Autodesk Inventor part; units mm, degrees
ref_plane "YZ Plane" through (0, 0, 0) normal (1, 0, 0) x (0, 1, 0)
ref_plane "XZ Plane" through (0, 0, 0) normal (0, 1, 0) x (-1, 0, 0)
ref_plane "XY Plane" through (0, 0, 0) normal (0, 0, 1) x (1, 0, 0)
sketch "Sketch1" plane through (0, 0, 0) normal (0, 0, 1) x (1, 0, 0)
  line L0 (17.35, -13.5) -> (-17.35, -13.5)
  line L1 (-17.35, -13.5) -> (-17.35, 13.5)
  line L2 (-17.35, 13.5) -> (17.35, 13.5)
  line L3 (17.35, 13.5) -> (17.35, -13.5)
  line L4 (17.35, -13.5) -> (-17.35, 13.5) construction
  line L5 (-17.35, -13.5) -> (17.35, 13.5) construction
  point P0 (0, 0)
  dimension "d0" = 27
  dimension "d1" = 34.7
extrude "Extrusion1" add sketch "Sketch1" along normal blind 10
sketch "Sketch2" plane through (0, 0, 10) normal (0, 0, 1) x (1, 0, 0)
  line L0 (17.35, -6) -> (-17.35, -6)
  line L1 (-17.35, -6) -> (-17.35, 6)
  line L2 (-17.35, 6) -> (17.35, 6)
  line L3 (17.35, 6) -> (17.35, -6)
  line L4 (17.35, -6) -> (-17.35, 6) construction
  line L5 (-17.35, -6) -> (17.35, 6) construction
  point P0 (0, 0)
  point P1 (17.35, 13.5)
  dimension "d4" = 12
extrude "Extrusion2" cut sketch "Sketch2" against normal blind 5
sketch "Sketch3" plane through (0, 0, 0) normal (0, 0, -1) x (-1, 0, 0)
  point P0 (0, 0)
  point P1 (-7.5, 10)
  point P2 (-7.5, -10)
  point P3 (7.5, 10)
  point P4 (7.5, -10)
  dimension "d7" = 20
  dimension "d8" = 10
  dimension "d9" = 15
  dimension "d10" = 7.5
hole "Hole1" at (7.5, 10, 0) at (7.5, -10, 0) at (-7.5, 10, 0) at (-7.5, -10, 0) direction (0, 0, 1) diameter 2.459 depth 8.8 tip angle 118
properties part number "MGN12C" material "Stainless Steel"
CAD build for the part. Positions are in the model's coordinates, mm. A direction names the side the tool comes from. Round coordinates to 2 decimals unless told otherwise and drop trailing zeros. Order: outer loops, then holes, each group sorted by start corner. A loop starts at its lowest first (then second) coordinate and runs counter-clockwise, first axis right, second up. Notation, with made-up numbers: M 31.25,-33.75 L 61.25,-33.75 A22 cw 61.25,-17.75 Z; hole C 10.5,56 d3. An arc over 180 degrees is marked long. Use one line per item in the form item = value.
Q1. Which spindle directions (+Z, -Z, +X, -X, +Y, -Y) get a long thin tool onto all of the face, cutting with end or side? Do faces 1 (the flat face through (0, 6, 8)), 2 (the flat face through (0, 0, 0)), 3 (the cylindrical face through (-6.41, -9.43, 4.46)). Say none if no direction does.
Recorded:
face_1 = +Z, +X, -X
face_2 = -Z, +X, -X, +Y, -Y
face_3 = -Z
Q2. Flat gauge pin, fed straight in: P1, Ø3, axis at x = -8, y = 1, coming from the +Z side. Where does the tip first touch, or does it go through?
Recorded:
P1 = 5
Q3. Saw through at D-D on y = -5.5. Give the cut face in (x, z), then the cut area to 4 significant figures.
Recorded:
outline = M -17.35,0 L 17.35,0 L 17.35,5 L -17.35,5 Z
area = 173.5 mm^2
Q4. Saw through at A-A on z = 6.75. Give the cut face in (x, y), then the cut area to 3 significant figures.
Recorded:
outline = M -17.35,-13.5 L 17.35,-13.5 L 17.35,-6 L -17.35,-6 Z; M -17.35,6 L 17.35,6 L 17.35,13.5 L -17.35,13.5 Z; hole C -7.5,-10 d2.46; hole C -7.5,10 d2.46; hole C 7.5,-10 d2.46; hole C 7.5,10 d2.46
area = 502 mm^2
Q5. Two-plate mould, pull along Y, no slides. Class faces 4 (the flat face through (0, -13.5, 5)), 5 (the flat face through (-17.35, 0, 4)), 6 (the conical face through (-7.63, -10.17, 9.41)), 7 (the conical face through (7.37, 9.83, 9.41)): +Y half, -Y half, draft (parallel to the pull), parting line (faces both ways), or undercut.
Recorded:
face_4 = -Y half
face_5 = draft
face_6 = undercut
face_7 = undercut
Q6. Probe L1, parallel to Y at x = -7.5, z = 4.25; L2, parallel to Y at x = 7.5, z = 5.5; L3, parallel to X at y = -10, z = 6.5. List the from-to ranges inside material, lowest first.
Recorded:
L1 = -13.5 to -11.23, -8.77 to 8.77, 11.23 to 13.5
L2 = -13.5 to -11.23, -8.77 to -6, 6 to 8.77, 11.23 to 13.5
L3 = -17.35 to -8.73, -6.27 to 6.27, 8.73 to 17.35
Q7. Saw through at B-B on z = 1. Give the cut face in (x, y).
Recorded:
outline = M -17.35,-13.5 L 17.35,-13.5 L 17.35,13.5 L -17.35,13.5 Z; hole C -7.5,-10 d2.46; hole C -7.5,10 d2.46; hole C 7.5,-10 d2.46; hole C 7.5,10 d2.46
Q8. Saw through at C-C on x = -12. Give the cut face in (y, z), then the cut area to 3 significant figures.
Recorded:
outline = M -13.5,0 L 13.5,0 L 13.5,10 L 6,10 L 6,5 L -6,5 L -6,10 L -13.5,10 Z
area = 210 mm^2
